Autodesk Inventor part; units mm, degrees
ref_plane "YZ Plane" through (0, 0, 0) normal (1, 0, 0) x (0, 1, 0)
ref_plane "XZ Plane" through (0, 0, 0) normal (0, 1, 0) x (-1, 0, 0)
ref_plane "XY Plane" through (0, 0, 0) normal (0, 0, 1) x (1, 0, 0)
sketch "Boceto1" plane through (0, 0, 0) normal (0, 0, 1) x (1, 0, 0)
  line L0 (0.8523, 2.6189) -> (11.8523, 36.4189)
  line L1 (13.7541, 37.8) -> (52.7541, 37.8)
  line L2 (54.7541, 35.8) -> (54.7541, 2)
  line L3 (52.7541, 0) -> (2.7541, 0)
  arc A0 (13.7541, 37.8) -> (11.8523, 36.4189) centre (13.7541, 35.8) ccw
  arc A1 (54.7541, 35.8) -> (52.7541, 37.8) centre (52.7541, 35.8) ccw
  arc A2 (52.7541, 0) -> (54.7541, 2) centre (52.7541, 2) ccw
  arc A3 (0.8523, 2.6189) -> (2.7541, 0) centre (2.7541, 2) ccw
  point P0 (0, 0)
  point P1 (12.3018, 37.8)
  point P2 (54.7541, 37.8)
  point P3 (54.7541, 0)
  dimension "d3" = 2
  dimension "d6" = 33.8
  dimension "d7" = 39
  dimension "d8" = 50
extrude "Extrusión1" add sketch "Boceto1" along normal blind 0.75
properties part number "VentanaLateralDelantera"
Model file for the job. Use its own axes, mm. Give positions to 0.01 mm unless a question says otherwise; leave off trailing zeros. Write each loop counter-clockwise with the first axis right and the second up, starting at its lowest first coordinate (ties: lowest second). Pieces come first, ordered by that corner, then holes. Notation, with made-up numbers: M 68,35.5 L 105,35.5 A7 ccw 105,44.5 Z; hole C 43.5,11.25 d7. An arc over 180 degrees is marked long. One line per item, written item: value. Start each with the question number.
Q1. Saw through at A-A, the plane z = 0.25. Write the cut outline in (x, y), plus the area to 3 significant figures.
Q2. Probe probe 1 along X at (y, z) = (33.5, 0.65); probe 2 along X at (y, z) = (14.5, 0.15). List the from-to ranges inside material, lowest first. Write a range as [from, to].
Q3. Saw through at C-C, the plane x = 6. Write the cut outline in (y, z).
Q4. Saw through at B-B, the plane y = 29.5. Write the cut outline in (x, z).
Output values:
1. outline: M 0.85,2.62 A2 ccw 2.75,0 L 52.75,0 A2 ccw 54.75,2 L 54.75,35.8 A2 ccw 52.75,37.8 L 13.75,37.8 A2 ccw 11.85,36.42 Z
1. area: 1,830 mm²
2. probe 1: x = [10.9, 54.75]
2. probe 2: x = [4.72, 54.75]
3. outline: M 0,0 L 18.44,0 L 18.44,0.75 L 0,0.75 Z
4. outline: M 9.6,0 L 54.75,0 L 54.75,0.75 L 9.6,0.75 Z
